Part model, mm, in its own coordinate system. A direction names the side the tool comes from. Coordinates: 2 decimals unless noted, no trailing zeros. Write each loop counter-clockwise with the first axis right and the second up, starting at its lowest first coordinate (ties: lowest second). Pieces come first, ordered by that corner, then holes. Notation, with made-up numbers: (-15, 88) -> (-2, 88) arc R23 cw to (-2, 125) -> close; hole circle Ø1 at (72, -19). An arc over 180 degrees is marked (long way). One line per question, with ' | ' between items. Start each with the question number.
Item 1: Saw through at D-D (x = 42.5). List the corners of the cut face in (y, z), and give its area (3 significant figures).
Item 2: Saw through at A-A (z = -5.5). List the corners of the cut face in (x, y), and give its area (3 significant figures).
Item 3: Saw through at B-B (x = -24). List the corners of the cut face in (y, z).
Item 4: 3-axis set-ups, long thin cutter, end or side, ignore diameter. For faces 1 (the flat face through (-22.39, 0.99, -41.62)), 2 (the flat face through (48.7, 1, 1)): which of +Z, -Z, +X, -X, +Y, -Y reach the whole face in a straight line?
Item 5: Saw through at C-C (z = -39). List the corners of the cut face in (x, y).
Item 6: Pin check, flat tips, straight feed: pin 1 (5 mm diameter, centred on x = 16.5, z = -1, fed in from +Y); pin 2 (0.8 mm diameter, centred on y = 2.5, z = 25, fed in from +X); pin 3 (1 mm diameter, centred on x = -22.5, y = 0.5, fed in from -Z); pin 4 (0.8 mm diameter, centred on x = 0, y = 2.5, fed in from -Z). Stop position of each tip, or through.
Item 7: Probe probe 1 along X at (y, z) = (0.8, 2); probe 2 along X at (y, z) = (2.3, 44.5); probe 3 along Z at (x, y) = (38, 0.1). List the from-to ranges inside material, lowest first. Write a range as [from, to].
Item 8: Two-plate mould, pull along X, no slides. Class faces 3 (the cylindrical face through (47.2, 0.99, -48.57)), 4 (the flat face through (47, 2.4, 23)), 5 (the cylindrical face through (-0.275, 0.986, -24.128)): pulls with the +X half, pulls with the -X half, needs draft (parallel to the pull), parting line crosses it, or undercut.
from build123d import *

# Parameters (mm, degrees)
GRUNDK_RPER_DEPTH  = 2
L_FTUNGEN_DEPTH    = 2
SKIZZE4_W          = 2
SKIZZE4_H          = 69
STREBE_DEPTH       = 1
STREBE_AU_EN_DEPTH = 0.4


with BuildPart() as part:
    # Skizze2 → Grundkörper (new body)
    with BuildSketch(Plane(origin=(0, 0, 0), x_dir=(1, 0, 0), z_dir=(0, 1, 0))):
        with BuildLine():
            Line((-43.7, 50), (-28, 50))
            Line((-28, 50), (-16.61985221, 33))
            ThreePointArc((-16.61985221, 33), (0, 24.125669082), (16.61985221, 33))
            Line((16.61985221, 33), (28, 50))
            Line((28, 50), (43.7, 50))
            ThreePointArc((43.7, 50), (47.235533906, 48.535533906), (48.7, 45))
            Line((48.7, 45), (48.7, -49))
            Line((48.7, -49), (-48.7, -49))
            Line((-48.7, -49), (-48.7, 45))
            ThreePointArc((-48.7, 45), (-47.235533906, 48.535533906), (-43.7, 50))
        make_face()
    extrude(amount=GRUNDK_RPER_DEPTH)

    # Skizze3 → Lüftungen (cut)
    with BuildSketch(Plane(origin=(0, 2, 0), x_dir=(1, 0, 0), z_dir=(0, 1, 0))):
        with BuildLine():
            Line((-39.25, 15), (-5.75, 15))
            ThreePointArc((-5.75, 15), (-4.335786438, 14.414213562), (-3.75, 13))
            Line((-3.75, 13), (-3.75, 9))
            ThreePointArc((-3.75, 9), (-4.335786438, 7.585786438), (-5.75, 7))
            Line((-5.75, 7), (-39.25, 7))
            ThreePointArc((-39.25, 7), (-40.664213562, 7.585786438), (-41.25, 9))
            Line((-41.25, 9), (-41.25, 13))
            ThreePointArc((-41.25, 13), (-40.664213562, 14.414213562), (-39.25, 15))
        make_face()
        with BuildLine():
            Line((3.75, 13), (3.75, 9))
            ThreePointArc((3.75, 9), (4.335786438, 7.585786438), (5.75, 7))
            Line((5.75, 7), (39.25, 7))
            ThreePointArc((39.25, 7), (40.664213562, 7.585786438), (41.25, 9))
            Line((41.25, 9), (41.25, 13))
            ThreePointArc((41.25, 13), (40.664213562, 14.414213562), (39.25, 15))
            Line((39.25, 15), (5.75, 15))
            ThreePointArc((5.75, 15), (4.335786438, 14.414213562), (3.75, 13))
        make_face()
        with BuildLine():
            Line((3.75, 1), (3.75, -3))
            ThreePointArc((3.75, -3), (4.335786438, -4.414213562), (5.75, -5))
            Line((5.75, -5), (39.25, -5))
            ThreePointArc((39.25, -5), (40.664213562, -4.414213562), (41.25, -3))
            Line((41.25, -3), (41.25, 1))
            ThreePointArc((41.25, 1), (40.664213562, 2.414213562), (39.25, 3))
            Line((39.25, 3), (5.75, 3))
            ThreePointArc((5.75, 3), (4.335786438, 2.414213562), (3.75, 1))
        make_face()
        with BuildLine():
            Line((3.75, -11), (3.75, -15))
            ThreePointArc((3.75, -15), (4.335786438, -16.414213562), (5.75, -17))
            Line((5.75, -17), (39.25, -17))
            ThreePointArc((39.25, -17), (40.664213562, -16.414213562), (41.25, -15))
            Line((41.25, -15), (41.25, -11))
            ThreePointArc((41.25, -11), (40.664213562, -9.585786438), (39.25, -9))
            Line((39.25, -9), (5.75, -9))
            ThreePointArc((5.75, -9), (4.335786438, -9.585786438), (3.75, -11))
        make_face()
        with BuildLine():
            Line((3.75, -23), (3.75, -27))
            ThreePointArc((3.75, -27), (4.335786438, -28.414213562), (5.75, -29))
            Line((5.75, -29), (39.25, -29))
            ThreePointArc((39.25, -29), (40.664213562, -28.414213562), (41.25, -27))
            Line((41.25, -27), (41.25, -23))
            ThreePointArc((41.25, -23), (40.664213562, -21.585786438), (39.25, -21))
            Line((39.25, -21), (5.75, -21))
            ThreePointArc((5.75, -21), (4.335786438, -21.585786438), (3.75, -23))
        make_face()
        with BuildLine():
            Line((3.75, -35), (3.75, -39))
            ThreePointArc((3.75, -39), (4.335786438, -40.414213562), (5.75, -41))
            Line((5.75, -41), (39.25, -41))
            ThreePointArc((39.25, -41), (40.664213562, -40.414213562), (41.25, -39))
            Line((41.25, -39), (41.25, -35))
            ThreePointArc((41.25, -35), (40.664213562, -33.585786438), (39.25, -33))
            Line((39.25, -33), (5.75, -33))
            ThreePointArc((5.75, -33), (4.335786438, -33.585786438), (3.75, -35))
        make_face()
        with BuildLine():
            Line((-41.25, 1), (-41.25, -3))
            ThreePointArc((-41.25, -3), (-40.664213562, -4.414213562), (-39.25, -5))
            Line((-39.25, -5), (-5.75, -5))
            ThreePointArc((-5.75, -5), (-4.335786438, -4.414213562), (-3.75, -3))
            Line((-3.75, -3), (-3.75, 1))
            ThreePointArc((-3.75, 1), (-4.335786438, 2.414213562), (-5.75, 3))
            Line((-5.75, 3), (-39.25, 3))
            ThreePointArc((-39.25, 3), (-40.664213562, 2.414213562), (-41.25, 1))
        make_face()
        with BuildLine():
            Line((-41.25, -11), (-41.25, -15))
            ThreePointArc((-41.25, -15), (-40.664213562, -16.414213562), (-39.25, -17))
            Line((-39.25, -17), (-5.75, -17))
            ThreePointArc((-5.75, -17), (-4.335786438, -16.414213562), (-3.75, -15))
            Line((-3.75, -15), (-3.75, -11))
            ThreePointArc((-3.75, -11), (-4.335786438, -9.585786438), (-5.75, -9))
            Line((-5.75, -9), (-39.25, -9))
            ThreePointArc((-39.25, -9), (-40.664213562, -9.585786438), (-41.25, -11))
        make_face()
        with BuildLine():
            Line((-41.25, -23), (-41.25, -27))
            ThreePointArc((-41.25, -27), (-40.664213562, -28.414213562), (-39.25, -29))
            Line((-39.25, -29), (-5.75, -29))
            ThreePointArc((-5.75, -29), (-4.335786438, -28.414213562), (-3.75, -27))
            Line((-3.75, -27), (-3.75, -23))
            ThreePointArc((-3.75, -23), (-4.335786438, -21.585786438), (-5.75, -21))
            Line((-5.75, -21), (-39.25, -21))
            ThreePointArc((-39.25, -21), (-40.664213562, -21.585786438), (-41.25, -23))
        make_face()
        with BuildLine():
            Line((-41.25, -35), (-41.25, -39))
            ThreePointArc((-41.25, -39), (-40.664213562, -40.414213562), (-39.25, -41))
            Line((-39.25, -41), (-5.75, -41))
            ThreePointArc((-5.75, -41), (-4.335786438, -40.414213562), (-3.75, -39))
            Line((-3.75, -39), (-3.75, -35))
            ThreePointArc((-3.75, -35), (-4.335786438, -33.585786438), (-5.75, -33))
            Line((-5.75, -33), (-39.25, -33))
            ThreePointArc((-39.25, -33), (-40.664213562, -33.585786438), (-41.25, -35))
        make_face()
    extrude(amount=-L_FTUNGEN_DEPTH, mode=Mode.SUBTRACT)

    # Skizze4 → Strebe (add)
    with BuildSketch(Plane(origin=(0, 2, 0), x_dir=(1, 0, 0), z_dir=(0, 1, 0))):
        with Locations((0, -12.5)):
            Rectangle(SKIZZE4_W, SKIZZE4_H)
    extrude(amount=STREBE_DEPTH)

    # Skizze5 → Strebe außen (add)
    with BuildSketch(Plane(origin=(0, 2, 0), x_dir=(1, 0, 0), z_dir=(0, 1, 0))):
        Polygon((-48.7, 45), (-46.7, 45), (-46.7, -47), (46.7, -47), (46.7, 45), (48.7, 45), (48.7, -49), (-48.7, -49), align=None)
    extrude(amount=STREBE_AU_EN_DEPTH)


solid = part.part
From the geometry:
1) outline: (0, -50) -> (2, -50) -> (2, 47) -> (2.4, 47) -> (2.4, 49) -> (0, 49) -> close | area: 199 mm2
2) outline: (-48.7, 0) -> (48.7, 0) -> (48.7, 2.4) -> (46.7, 2.4) -> (46.7, 2) -> (1, 2) -> (1, 3) -> (-1, 3) -> (-1, 2) -> (-46.7, 2) -> (-46.7, 2.4) -> (-48.7, 2.4) -> close | area: 198 mm2
3) outline: (0, -44.02) -> (2, -44.02) -> (2, -15) -> (0, -15) -> close; (0, -7) -> (2, -7) -> (2, -3) -> (0, -3) -> close; (0, 5) -> (2, 5) -> (2, 9) -> (0, 9) -> close; (0, 17) -> (2, 17) -> (2, 21) -> (0, 21) -> close; (0, 29) -> (2, 29) -> (2, 33) -> (0, 33) -> close; (0, 41) -> (2, 41) -> (2, 47) -> (2.4, 47) -> (2.4, 49) -> (0, 49) -> close
4) face 1: -Z, +Y, -Y | face 2: +Z, -Z, +X, +Y, -Y
5) outline: (-48.7, 0) -> (-20.64, 0) -> (-20.64, 2) -> (-46.7, 2) -> (-46.7, 2.4) -> (-48.7, 2.4) -> close; (20.64, 0) -> (48.7, 0) -> (48.7, 2.4) -> (46.7, 2.4) -> (46.7, 2) -> (20.64, 2) -> close
6) pin 1: y = 2 | pin 2: x = 48.7 | pin 3: z = -42.53 | pin 4: z = -22
7) probe 1: [-48.7, -41.25], [-3.75, 3.75], [41.25, 48.7] | probe 2: [-48.7, -46.7], [-1, 1], [46.7, 48.7] | probe 3: [-50, -15], [-7, -3], [5, 9], [17, 21], [29, 33], [41, 49]
8) face 3: pulls with the +X half | face 4: needs draft | face 5: undercut
